from build123d import *

# Parameters (mm, degrees)
F0_W     = 100
F0_H     = 80
F0_R     = 20
F1_DEPTH = 44
F3_DEPTH = 20


with BuildPart() as f1:
    # F0 (on Top) → F1 (new body)
    with BuildSketch(Plane.XY):
        Rectangle(F0_W, F0_H)
        Circle(F0_R, mode=Mode.SUBTRACT)
    extrude(amount=F1_DEPTH)

    # F2 (on face) → F3 (cut)
    with BuildSketch(Plane.XY.offset(44)):
        with BuildLine():
            Line((50, -40), (50, 40))
            Line((50, 40), (-14, 40))
            Line((-14, 40), (-2.8849574507, 19.7908317285))
            ThreePointArc((-2.8849574507, 19.7908317285), (13.0824472287, 15.1277749358), (20, 0))
            ThreePointArc((20, 0), (18.7534067701, -6.9505204492), (15.1690265486, -13.0345937247))
            Line((15.1690265486, -13.0345937247), (30, -40))
            Line((30, -40), (50, -40))
        make_face()
    extrude(amount=-F3_DEPTH, mode=Mode.SUBTRACT)


solid = f1.part
Build history of the part. All positions in model axes, mm. A direction names the side the tool comes from. Give positions to 0.01 mm unless a question says otherwise; leave off trailing zeros. Write each loop counter-clockwise with the first axis right and the second up, starting at its lowest first coordinate (ties: lowest second). Pieces come first, ordered by that corner, then holes. Notation, with made-up numbers: (77.25, 59) - (88.25, 59) arc R23 ccw to (88.25, 69) - close; hole circle Ø8 at (3.25, 54.5). An arc over 180 degrees is marked (long way). Use one line per item in the form item = value. Start each with the question number.
1. Drop flat-ended pins along their axis: pin 1 Ø3 at (y, z) = (-15.5, 28.5) entering from +X; pin 2 Ø1 at (x, z) = (-10.5, 32.5) entering from +Y. Give the stop position or say it passes through.
2. Probe line 1 (Y direction, x = 0, z = 14); line 2 (X direction, y = 0, z = 17.5); line 3 (Z direction, x = 38, y = -3.5). List the from-to ranges inside material, lowest first. Write a range as [from, to].
3. Band-saw the part on C-C on z = 36. Write the cut outline in (x, y), plus the area to 3 significant figures.
4. Band-saw the part on D-D on y = 23. Write the cut outline in (x, z), plus the area to 3 significant figures.
5. Band-saw the part on B-B on y = 14.5. Write the cut outline in (x, z), plus the area to 3 significant figures.
6. 3-axis set-ups, long thin cutter, end or side, ignore diameter. For faces 5 (the face through (-19, -8, 44)), 6 (the face through (-8.5, 30, 34.1)): which of +Z, -Z, +X, -X, +Y, -Y reach the whole face in a straight line?
7. Band-saw the part on A-A on x = 0. Write the cut outline in (y, z).
8. Two-plate mould, pull along X, no slides. Class faces 1 (the face through (-16, -12, 17)), 2 (the face through (50, -1, 12)), 3 (the face through (-12, 40, 17)), 4 (the face through (-50, -1, 22)): released by +X, released by -X, zero draft, split by the parting line, or undercut.
Conclusion:
q1.pin_1 = 17.35
q1.pin_2 = 34.55
q2.line_1 = [-40, -20], [20, 40]
q2.line_2 = [-50, -20], [20, 50]
q2.line_3 = [0, 24]
q3.outline = (-50, -40) - (30, -40) - (15.17, -13.03) arc R20 cw (long way) to (-2.88, 19.79) - (-14, 40) - (-50, 40) - close
q3.area = 3,740 mm²
q4.outline = (-50, 0) - (50, 0) - (50, 24) - (-4.65, 24) - (-4.65, 44) - (-50, 44) - close
q4.area = 3,310 mm²
q5.outline = (-50, 0) - (-13.77, 0) - (-13.77, 44) - (-50, 44) - close; (13.77, 0) - (50, 0) - (50, 24) - (13.77, 24) - close
q5.area = 2,460 mm²
q6.face_5 = +Z, +X, -X, +Y, -Y
q6.face_6 = +Z, +X, +Y
q7.outline = (-40, 0) - (-20, 0) - (-20, 44) - (-40, 44) - close; (20, 0) - (40, 0) - (40, 24) - (20, 24) - close
q8.face_1 = undercut
q8.face_2 = released by +X
q8.face_3 = zero draft
q8.face_4 = released by -X
